Part print with two shaded views. Sizes in mm from the minimum x, y, z corner. A direction names the side the tool comes from. Round coordinates to 2 decimals unless told otherwise and drop trailing zeros. Write each loop counter-clockwise with the first axis right and the second up, starting at its lowest first coordinate (ties: lowest second). Pieces come first, ordered by that corner, then holes. Notation, with made-up numbers: (75.25, 37.5) - (90.25, 37.5) arc R14 ccw to (90.25, 57.5) - close; hole circle Ø9 at (86.5, -16). An arc over 180 degrees is marked (long way). Answer as a JSON object with one key per item and string values. Group by question number.
Item 1: Which spindle directions (+Z, -Z, +X, -X, +Y, -Y) get a long thin tool onto all of the face, cutting with end or side? Do the marked faces 1, 2, 3 and 4. Say none if no direction does.
Item 2: Probe line 1 (X direction, y = 45.5, z = 97); line 2 (Y direction, x = 39, z = 35); line 3 (Z direction, x = 96, y = 27). List the from-to ranges inside material, lowest first. Write a range as from..to.
Item 3: Slice it at B-B, the plane x = 82. List the corners of the cut face in (y, z).
Item 4: Flat gauge pins, fed straight in: pin 1 (2 mm diameter, centred on x = 31, y = 10.5, fed in from -Z); pin 2 (4 mm diameter, centred on y = 38, z = 91, fed in from -X); pin 3 (2 mm diameter, centred on x = 116.5, y = 41.5, fed in from -Z). Where does each tip first touch, or does it go through?
Item 5: Slice it at C-C, the plane y = 48.5. List the corners of the cut face in (x, z), then the cut area to 3 significant figures.
Item 6: Slice it at A-A, the plane z = 74. List the corners of the cut face in (x, y) (1 decimal), then the cut area to 3 significant figures.
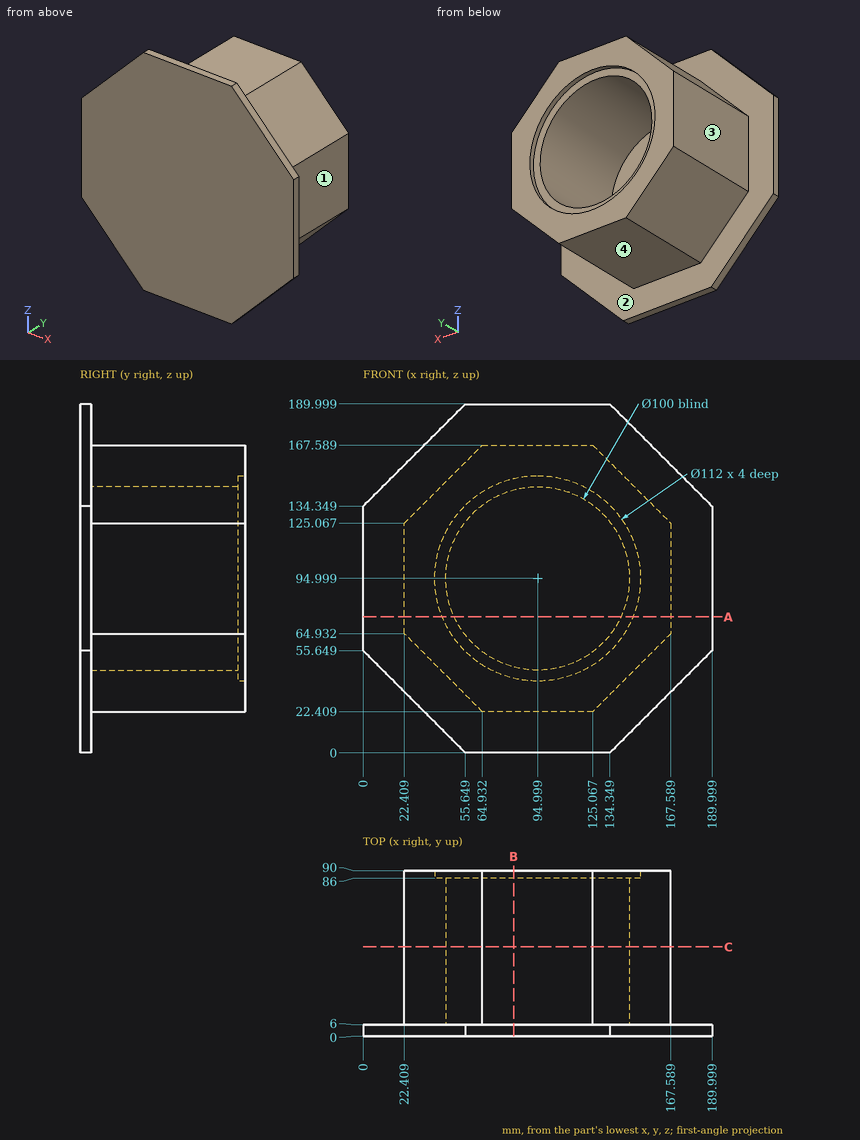
Geometry says:
{
 "1": {"face 1": "+Z, -Z, +X, +Y", "face 2": "+Y", "face 3": "+Z, -Z, -X, +Y", "face 4": "-Z, +X, -X, +Y"},
 "2": {"line 1": "x = 22.41..45.04, 144.96..167.59", "line 2": "y = 0..6", "line 3": "z = 22.41..45.01, 144.99..167.59"},
 "3": {"outline": "(0, 0) - (6, 0) - (6, 22.41) - (90, 22.41) - (90, 40.53) - (86, 40.53) - (86, 46.72) - (6, 46.72) - (6, 143.28) - (86, 143.28) - (86, 149.47) - (90, 149.47) - (90, 167.59) - (6, 167.59) - (6, 190) - (0, 190) - close"},
 "4": {"pin 1": "stops at z = 55.34", "pin 2": "stops at x = 22.41", "pin 3": "stops at z = 22.41"},
 "5": {"outline": "(22.41, 64.93) - (64.93, 22.41) - (125.07, 22.41) - (167.59, 64.93) - (167.59, 125.07) - (125.07, 167.59) - (64.93, 167.59) - (22.41, 125.07) - close; hole circle Ø100 at (95, 95)", "area": "9,610 mm^2"},
 "6": {"outline": "(0, 0) - (190, 0) - (190, 6) - (167.6, 6) - (167.6, 90) - (146.9, 90) - (146.9, 86) - (140.4, 86) - (140.4, 6) - (49.6, 6) - (49.6, 86) - (43.1, 86) - (43.1, 90) - (22.4, 90) - (22.4, 6) - (0, 6) - close", "area": "5,660 mm^2"}
}
